Read the model definition and answer for the solid it produces. Units are mm, in the model's axes. Face numbers are marked on the shaded views. Give positions to 0.01 mm unless a question says otherwise; leave off trailing zeros. Write each loop counter-clockwise with the first axis right and the second up, starting at its lowest first coordinate (ties: lowest second). Pieces come first, ordered by that corner, then holes.
Autodesk Inventor part; units mm, degrees
ref_plane "YZ Plane" through (0, 0, 0) normal (1, 0, 0) x (0, 1, 0)
ref_plane "XZ Plane" through (0, 0, 0) normal (0, 1, 0) x (-1, 0, 0)
ref_plane "XY Plane" through (0, 0, 0) normal (0, 0, 1) x (1, 0, 0)
sketch "Sketch1" plane through (0, 0, 0) normal (0, 0, 1) x (1, 0, 0)
  line L0 (0, 0) -> (19, 0)
  line L1 (19, 0) -> (19, 15)
  line L2 (19, 15) -> (0, 15)
  line L3 (0, 15) -> (0, 0)
  point P0 (9.5, 15)
  dimension "d0" = 19
  dimension "d1" = 15
extrude "Extrusion1" add sketch "Sketch1" along normal blind 3
sketch "Sketch2" plane through (0, 0, 3) normal (0, 0, 1) x (1, 0, 0)
  line L0 (19, 15) -> (0, 15)
  circle A0 centre (9.5, 13) radius 1
  point P0 (0, 0)
  point P1 (9.5, 15)
  dimension "d4" = 2
  dimension "d5" = 2
extrude "Extrusion2" add sketch "Sketch2" along normal blind 1.5
sketch "Sketch6" plane through (9.5, 13, 4.5) normal (0, 0, 1) x (1, 0, 0)
  circle A0 centre (0, 0) radius 1
  line L0 (2, -1) -> (-2, -1)
  line L1 (-2, -1) -> (-2, 1)
  line L2 (-2, 1) -> (2, 1)
  line L3 (2, 1) -> (2, -1)
  line L4 (2, -1) -> (-2, 1) construction
  line L5 (-2, -1) -> (2, 1) construction
  point P0 (-9.5, -13)
  dimension "d13" = 4
extrude "Extrusion5" add sketch "Sketch6" along normal blind 47
sketch "Sketch7" plane through (9.5, 13, 51.5) normal (0, 0, 1) x (1, 0, 0)
  circle A0 centre (0, 0) radius 1
  line L0 (-9.5, -13) -> (9.5, -13)
  line L1 (9.5, -13) -> (9.5, 2)
  line L2 (9.5, 2) -> (-9.5, 2)
  line L3 (-9.5, 2) -> (-9.5, -13)
  arc A1 (0, -1) -> (0, 1) centre (0, 0) ccw
  arc A2 (0, 1) -> (0, -1) centre (0, 0) ccw
extrude "Extrusion6" add sketch "Sketch7" along normal blind 4 contours A0 | L3 L2 L1 L0
fillet "Fillet2" radius 1 4 edges at (19, 0, 1.5) (19, 15, 1.5) (0, 0, 1.5) (0, 15, 1.5)
fillet "Fillet3" radius 2 4 edges at (19, 0, 53.5) (19, 15, 53.5) (0, 0, 53.5) (0, 15, 53.5)
extrude "Extrusion10" add sketch "Sketch6" against normal up to surface (1.5 mm away) contours A0 L2 L3 L0 | A0 L0 L1 L2
sketch "Sketch13" plane through (0, 0, 3) normal (0, 0, 1) x (1, 0, 0)
  line L0 (11.5, 12) -> (7.5, 12)
  line L1 (7.5, 12) -> (7.5, 14)
  line L2 (7.5, 14) -> (11.5, 14)
  line L3 (11.5, 14) -> (11.5, 12)
  arc A0 (1, 15) -> (0, 14) centre (1, 14) ccw
  line L4 (0, 14) -> (0, 1)
  arc A1 (0, 1) -> (1, 0) centre (1, 1) ccw
  line L5 (1, 0) -> (18, 0)
  arc A2 (18, 0) -> (19, 1) centre (18, 1) ccw
  line L6 (19, 1) -> (19, 14)
  arc A3 (19, 14) -> (18, 15) centre (18, 14) ccw
  line L7 (18, 15) -> (1, 15)
  line L8 (4.5, 10.2) -> (14.7, 10.2)
  line L9 (14.7, 10.2) -> (14.7, 0)
  line L10 (14.7, 0) -> (4.5, 0)
  line L11 (4.5, 0) -> (4.5, 10.2)
  point P0 (0, 0)
  point P1 (14.7, 0)
  dimension "d67" = 10.2
  dimension "d68" = 10.2
  dimension "d69" = 4.5
extrude "Extrusion12" cut sketch "Sketch13" against normal blind 1 contours L11 L8 L9 L5
ref_plane "Work Plane1" through (0, 0, 16) normal (0, 0, 1) x (1, 0, 0)
sketch "Sketch14" plane through (0, 0, 16) normal (0, 0, 1) x (1, 0, 0)
  line L0 (4.5, 0) -> (4.5, 10.2)
  line L1 (4.5, 10.2) -> (14.7, 10.2)
  line L2 (14.7, 10.2) -> (14.7, 0)
  line L3 (14.7, 0) -> (18, 0)
  arc A0 (18, 0) -> (19, 1) centre (18, 1) ccw
  line L4 (19, 1) -> (19, 14)
  arc A1 (19, 14) -> (18, 15) centre (18, 14) ccw
  line L5 (18, 15) -> (1, 15)
  arc A2 (1, 15) -> (0, 14) centre (1, 14) ccw
  line L6 (0, 14) -> (0, 1)
  arc A3 (0, 1) -> (1, 0) centre (1, 1) ccw
  line L7 (1, 0) -> (4.5, 0)
  line L8 (11.5, 12) -> (7.5, 12)
  line L9 (7.5, 12) -> (7.5, 14)
  line L10 (7.5, 14) -> (11.5, 14)
  line L11 (11.5, 14) -> (11.5, 12)
  line L12 (4.5, 0) -> (4.5, 10.2)
  line L13 (14.7, 0) -> (4.5, 0)
  line L14 (14.7, 10.2) -> (14.7, 0)
  line L15 (4.5, 10.2) -> (14.7, 10.2)
  point P0 (0, 0)
extrude "Extrusion13" add sketch "Sketch14" along normal blind 3
sketch "Sketch15" plane through (0, 0, 19) normal (0, 0, 1) x (1, 0, 0)
  line L0 (4.5, 0) -> (4.5, 10.2)
  line L1 (14.7, 0) -> (4.5, 0)
  line L2 (14.7, 10.2) -> (14.7, 0)
  line L3 (4.5, 10.2) -> (14.7, 10.2)
  point P0 (0, 0)
  point P1 (9.6, 5.1)
hole "Hole1" at (9.6, 5.1, 19) direction (0, 0, -1) diameter 3.242 end through all
extrude "Extrusion14" cut sketch "Sketch14" along normal blind 1 contours L0 L1 L2 L13
sketch "Sketch16" plane through (9.5, 13, 55.5) normal (0, 0, 1) x (1, 0, 0)
  circle A0 centre (0.1, -7.9) radius 1.621
  point P0 (-9.5, -13)
extrude "Extrusion15" cut sketch "Sketch16" against normal up to surface (4 mm away)
properties part number "Crystal-Cut10x10-screwM4"
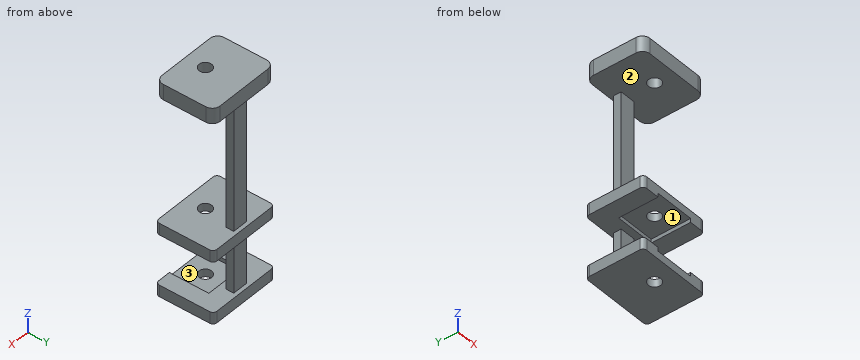
Item 1: Section B-B (y = 5.1) is taken. Give the number of separate pieces and of enclosed holes in the cut face, and give its area (3 significant figures).
Result set:
separate pieces: 6
enclosed holes: 0
area: 144 mm2
Item 2: Section C-C (y = 2.5) is taken. Write down the section's boundary in (x, z), and give its area (3 significant figures).
Result set:
outline: (0, 0) - (19, 0) - (19, 3) - (14.7, 3) - (14.7, 2) - (4.5, 2) - (4.5, 3) - (0, 3) - close; (0, 16) - (4.5, 16) - (4.5, 17) - (14.7, 17) - (14.7, 16) - (19, 16) - (19, 19) - (0, 19) - close; (0, 51.5) - (19, 51.5) - (19, 55.5) - (0, 55.5) - close
area: 170 mm2
Item 3: Find the intervals of material crossed by line 1 along Z through (x, y) = (15.25, 1); line 2 along Z through (x, y) = (6, 4); line 3 along X through (y, z) = (5.1, 17.5), in increasing order.
Result set:
line 1: z = 0 to 3, 16 to 19, 51.5 to 55.5
line 2: z = 0 to 2, 17 to 19, 51.5 to 55.5
line 3: x = 0 to 7.98, 11.22 to 19
Item 4: Each of these flat-tipped pins is pushed along its axis until it touches: pin 1 Ø4.5 at (x, z) = (10.5, 31) entering from +Y; pin 2 Ø1.2 at (x, z) = (10, 41) entering from -Y; pin 3 Ø2 at (y, z) = (12.5, 8) entering from -X. Where does it stop, or does it pass through?
Result set:
pin 1: stops at y = 14
pin 2: stops at y = 12
pin 3: stops at x = 7.5
Item 5: Determine the mould class of the marked faces 1, 2 and 3 for opening direction X: pulls with the +X half, pulls with the -X half, needs draft (parallel to the pull), parting line crosses it, or undercut.
Result set:
face 1: undercut
face 2: needs draft
face 3: undercut
Item 6: Section A-A (x = 2.5) is taken. Write down the section's boundary in (y, z).
Result set:
outline: (0, 0) - (15, 0) - (15, 3) - (0, 3) - close; (0, 16) - (15, 16) - (15, 19) - (0, 19) - close; (0, 51.5) - (15, 51.5) - (15, 55.5) - (0, 55.5) - close
